Could you check a few things on this model? Use its own coordinates, in mm. A direction names the side the tool comes from. Give positions to 0.01 mm unless a question says otherwise; leave off trailing zeros. Loops run counter-clockwise (first coordinate to the right, second up) from the corner with the lowest first, then second, coordinate; pieces in that order, holes last. Notation, with made-up numbers: M 17,85.25 L 64,85.25 A31 cw 64,114.25 Z; hole C 12.5,10 d6. An arc over 180 degrees is marked long. Write each question's results on one line, items separated by ' | '. Start each with the question number.
from build123d import *

# Parameters (mm, degrees)
SKETCH_2_R          = 1.5
SKETCH_2_R_2        = 9.5
EXTRUDE_1_DEPTH     = 4
CUT_EXTRUDE_1_DEPTH = 124.429075185
EXTRUDE_2_DEPTH     = 4
SKETCH_7_R          = 1.5
CUT_EXTRUDE_2_DEPTH = 155.008884812
CUT_EXTRUDE_5_DEPTH = 155.008884812
FILLET_4_R          = 3
FILLET_5_R          = 6
FILLET_6_R          = 10
CHAMFER_1_SIZE      = 20
CHAMFER_1_SIZE2     = 38.078865529


with BuildPart() as part:
    # 草图2 → 凸台-拉伸1 (new body)
    with BuildSketch(Plane(origin=(0, 0, 0), x_dir=(1, 0, 0), z_dir=(0, 1, 0))):
        Polygon((0, 0), (0, 60), (40, 93.908128514), (80, 60), (80, 0), (68, 0), (68, 42), (40, 54), (12, 42), (12, 0), align=None)
        with Locations(Location((6, 32, 0), (0, 0, 270))):
            Circle(SKETCH_2_R, mode=Mode.SUBTRACT)
        with Locations(Location((6, 8, 0), (0, 0, 270))):
            Circle(SKETCH_2_R, mode=Mode.SUBTRACT)
        with Locations(Location((40, 69, 0), (0, 0, 270))):
            Circle(SKETCH_2_R_2, mode=Mode.SUBTRACT)
        with Locations(Location((74, 8, 0), (0, 0, 90))):
            Circle(SKETCH_2_R, mode=Mode.SUBTRACT)
        with Locations(Location((74, 32, 0), (0, 0, 90))):
            Circle(SKETCH_2_R, mode=Mode.SUBTRACT)
    extrude(amount=EXTRUDE_1_DEPTH)

    # 草图4 → 切除-拉伸1 (cut, through all)
    with BuildSketch(Plane(origin=(0, 4, 0), x_dir=(1, 0, 0), z_dir=(0, 1, 0))):
        with BuildLine():
            Line((24.36723091, 80.656179931), (0, 60))
            Line((0, 60), (0, 0))
            Line((0, 0), (12, 0))
            Line((12, 0), (12, 42))
            Line((12, 42), (32.756034747, 50.895443463))
            ThreePointArc((32.756034747, 50.895443463), (21.23136653, 63.709593809), (24.36723091, 80.656179931))
        make_face()
    extrude(amount=-CUT_EXTRUDE_1_DEPTH, mode=Mode.SUBTRACT)

    # 草图6 → 凸台-拉伸2 (add)
    with BuildSketch(Plane(origin=(0, 4, 0), x_dir=(1, 0, 0), z_dir=(0, 1, 0))):
        with BuildLine():
            ThreePointArc((122, 55.435340034), (101, 44), (80, 55.435340034))
            Line((80, 55.435340034), (80, 0))
            Line((80, 0), (122, 0))
            Line((122, 0), (122, 55.435340034))
        make_face()
    extrude(amount=-EXTRUDE_2_DEPTH)

    # 草图7 → 切除-拉伸2 (cut, through all)
    with BuildSketch(Plane(origin=(0, 4, 0), x_dir=(1, 0, 0), z_dir=(0, 1, 0))):
        with Locations(Location((91, 32, 0), (0, 0, 270))):
            Circle(SKETCH_7_R)
        with Locations(Location((74, 32, 0), (0, 0, 90))):
            Circle(SKETCH_7_R)
        with Locations(Location((74, 8, 0), (0, 0, 90))):
            Circle(SKETCH_7_R)
        with Locations(Location((111, 32, 0), (0, 0, 270))):
            Circle(SKETCH_7_R)
        with Locations(Location((111, 8, 0), (0, 0, 270))):
            Circle(SKETCH_7_R)
        with Locations(Location((91, 8, 0), (0, 0, 270))):
            Circle(SKETCH_7_R)
    extrude(amount=-CUT_EXTRUDE_2_DEPTH, mode=Mode.SUBTRACT)

    # 草图9 → 切除-拉伸5 (cut, through all)
    with BuildSketch(Plane(origin=(0, 4, 0), x_dir=(1, 0, 0), z_dir=(0, 1, 0))):
        Polygon((122, 30), (92, 0), (122, 0), align=None)
    extrude(amount=-CUT_EXTRUDE_5_DEPTH, mode=Mode.SUBTRACT)

    # 圆角4
    fillet_4_edges = [part.edges().sort_by_distance(p)[0] for p in [
        (122, 2, -30),
        (92, 2, 0),
    ]]
    fillet(fillet_4_edges, radius=FILLET_4_R)

    # 圆角5
    fillet_5_edges = [part.edges().sort_by_distance(p)[0] for p in [
        (122, 2, -55.435340034),
    ]]
    fillet(fillet_5_edges, radius=FILLET_5_R)

    # 圆角6
    # the kernel refuses this fillet: 10 mm, written as the material it takes off along each edge
    with BuildSketch(Plane(origin=(80, -11.580514233, -60), x_dir=(0, 0, 1), z_dir=(0, 1, 0))) as fillet_6_piece_1:
        with BuildLine():
            CenterArc((4.632705448, -9.999768488), FILLET_6_R, 90.389874902, 49.322073547)
            Line((-2.995326497, -3.5334613), (-3.147887136, -3.404135157))
            Line((-3.147887136, -3.404135157), (-0.152560639, 0.129326144))
            Line((-0.152560639, 0.129326144), (0, 0.2))
            ThreePointArc((0, 0.2), (2.282329983, 0.2), (4.563299057, 0.19999537))
            Line((4.563299057, 0.19999537), (4.564659966, 0))
        make_face()
    extrude(amount=27.161028465, mode=Mode.SUBTRACT)

    # 倒角1
    chamfer_1_edges = [part.edges().sort_by_distance(p)[0] for p in [
        (68, 2, -42),
    ]]
    chamfer_1_side = [part.faces().sort_by_distance(p)[0] for p in [
        (54, 2, -48),
    ]]
    chamfer(chamfer_1_edges, length=CHAMFER_1_SIZE, length2=CHAMFER_1_SIZE2, reference=chamfer_1_side[0])


solid = part.part
1) If we section it at A-A on x = 74: Write out the boundary of the cut face in (y, z).
2) Which directions (+Z, -Z, +X, -X, +Y, -Y) give clear straight access to the entire face, cutting with the end or side of a thin tool? Please do faces 5 (the face through (68, 2, -2)), 6 (the face through (79, 2, 0)), 7 (the face through (36.43, 1.97, -52.47)).
3) Thinking about a two-plate mould opening in X: for faces 1 (the face through (71, 0, -37)), 2 (the face through (72.513, 1.972, -7.805)), 3 (the face through (21.3, 2.03, -63.47)), 4 (the face through (107, 2, -15)), which applies, pulls with the +X half, pulls with the -X half, needs draft (parallel to the pull), parting line crosses it, or undercut?
4) I'm going to push flat-ended pins straight in: P1, Ø1.8, axis at x = 111, z = -32, coming from the -Y side; P2, Ø1, axis at y = 3.5, z = -40.5, coming from the -X side; P3, Ø1.2, axis at y = 2.5, z = -2.5, coming from the -X side; P4, Ø1, axis at y = 2, z = -56.5, coming from the +X side. Where does each tip first touch, or does it pass through?
5) If we section it at D-D on x = 111: Write out the boundary of the cut face in (y, z).
6) If we section it at C-C on z = -69: Write out the boundary of the cut face in (x, y), plus the area to 3 significant figures.
7) Please list where these lines run through material, in increasing order: line 1 (Z direction, x = 74, y = 1.45); line 2 (X direction, y = 1.3, z = -32); line 3 (Z direction, x = 91, y = 1.45). Write a range as from..to.
8) If we section it at B-B on y = 0.9: Write out the boundary of the cut face in (x, z), plus the area to 3 significant figures.
Calculated:
1) outline: M 0,-65.09 L 4,-65.09 L 4,-33.5 L 0,-33.5 Z; M 0,-30.5 L 4,-30.5 L 4,-9.5 L 0,-9.5 Z; M 0,-6.5 L 4,-6.5 L 4,0 L 0,0 Z
2) face 5: +Z, -X, +Y, -Y | face 6: +Z, +X, -X, +Y, -Y | face 7: +Z, +Y, -Y
3) face 1: needs draft | face 2: undercut | face 3: pulls with the -X half | face 4: pulls with the +X half
4) P1: passes through | P2: stops at x = 53.17 | P3: stops at x = 68 | P4: stops at x = 79.98
5) outline: M 0,-46.09 L 4,-46.09 L 4,-33.5 L 0,-33.5 Z; M 0,-30.5 L 4,-30.5 L 4,-19 L 0,-19 Z
6) outline: M 20.5,0 L 30.5,0 L 30.5,4 L 20.5,4 Z; M 49.5,0 L 69.38,0 L 69.38,4 L 49.5,4 Z | area: 120 mm2
7) line 1: z = -65.09..-33.5, -30.5..-9.5, -6.5..0 | line 2: x = 56.77..72.5, 75.5..89.5, 92.5..109.5, 112.5..122 | line 3: z = -46.09..-33.5, -30.5..-9.5, -6.5..-0.01
8) outline: M 24.37,-80.66 L 40,-93.91 L 76.47,-63 A10 ccw 80,-55.44 A25 cw 113.1,-47.12 A6 ccw 122,-41.87 L 122,-31.24 A3 ccw 121.12,-29.12 L 92.88,-0.88 A3 ccw 90.76,0 L 68,0 L 68,-3.92 L 49.62,-49.88 L 40,-54 L 32.76,-50.9 A19.5 ccw Z; hole C 40,-69 d19; hole C 74,-32 d3; hole C 74,-8 d3; hole C 91,-32 d3; hole C 91,-8 d3; hole C 111,-32 d3 | area: 3,870 mm2
